from build123d import *

# Parameters (mm, degrees)
SKETCH_1_R          = 1.3
SKETCH_1_W          = 7.4992
SKETCH_1_H          = 3.0001
SKETCH_1_W_2        = 4.9995
EXTRUDE_1_DEPTH     = 3
SKETCH_2_R          = 1.6
CUT_EXTRUDE_1_DEPTH = 57.708942736


with BuildPart() as part:
    # 草图1 → 凸台-拉伸1 (new body)
    with BuildSketch(Plane(origin=(0, 0, 0), x_dir=(-1, 0, 0), z_dir=(0, 0, -1))):
        with BuildLine():
            Line((-30.618171933, 0), (49.343510787, 0))
            ThreePointArc((49.343510787, 0), (55.343510787, 6), (49.343510787, 12))
            Line((49.343510787, 12), (-30.618171933, 12))
            ThreePointArc((-30.618171933, 12), (-36.618171933, 6), (-30.618171933, 0))
        make_face()
        with Locations(Location((49.343510787, 6, 0), (0, 0, 180))):
            Circle(SKETCH_1_R, mode=Mode.SUBTRACT)
        with Locations(Location((1.379286828, 6.00015, 0), (0, 0, 180))):
            Circle(SKETCH_1_R, mode=Mode.SUBTRACT)
        with Locations(Location((-30.611606698, 6.0001, 0), (0, 0, 180))):
            Circle(SKETCH_1_R, mode=Mode.SUBTRACT)
        with Locations((35.628693302, 5.99945)):
            Rectangle(SKETCH_1_W, SKETCH_1_H, mode=Mode.SUBTRACT)
        with Locations((-18.121556698, 5.99945)):
            Rectangle(SKETCH_1_W_2, SKETCH_1_H, mode=Mode.SUBTRACT)
    extrude(amount=-EXTRUDE_1_DEPTH)

    # 草图2 → 切除-拉伸1 (cut, through all)
    with BuildSketch(Plane.XY.offset(3)):
        with Locations((-49.343510787, 6)):
            Circle(SKETCH_2_R)
        with Locations((-1.379286828, 6.00015)):
            Circle(SKETCH_2_R)
    extrude(amount=-CUT_EXTRUDE_1_DEPTH, mode=Mode.SUBTRACT)


solid = part.part
Read the model definition and answer for the solid it produces. Units are mm, in the model's axes. A direction names the side the tool comes from. Coordinates: 2 decimals unless noted, no trailing zeros. Loops run counter-clockwise (first coordinate to the right, second up) from the corner with the lowest first, then second, coordinate; pieces in that order, holes last. Notation, with made-up numbers: (24.5, 7) -> (36.5, 7) arc R16 ccw to (36.5, 19) -> close; hole circle Ø10 at (52.5, 15.25). An arc over 180 degrees is marked (long way). Answer in a Markdown table with one row per item.
Item 1: For a pull along Y with two mould halves and no side action, classify faces 3 (the flat face through (20.621, 6, 1)), 4 (the cylindrical face through (36.617, 6.132, 1.479)), 5 (the flat face through (-10, 12, 1)) as released by +Y, released by -Y, zero draft, split by the parting line, or undercut.
Returned:
| item | result |
|---|---|
| face 3 | undercut |
| face 4 | split by the parting line |
| face 5 | released by +Y |
Item 2: A cutting plane is placed at B-B on z = 0.75. Determine the outline of the cut face in (x, y).
Returned:
| item | result |
|---|---|
| outline | (-49.34, 0) -> (30.62, 0) arc R6 ccw to (30.62, 12) -> (-49.34, 12) arc R6 ccw to start; hole circle Ø3.2 at (-49.34, 6); hole (-39.38, 4.5) -> (-31.88, 4.5) -> (-31.88, 7.5) -> (-39.38, 7.5) -> close; hole circle Ø3.2 at (-1.38, 6); hole (15.62, 4.5) -> (20.62, 4.5) -> (20.62, 7.5) -> (15.62, 7.5) -> close; hole circle Ø2.6 at (30.61, 6) |
Item 3: Straight lines are drawn through the part: line 1 along X through (y, z) = (5.75, 0.95); line 2 along X through (y, z) = (5, 0.2); line 3 along Y through (x, z) = (-37.5, 1.8). For each, find the intervals that lie inside material, in ascending order. Write a range as [from, to].
Returned:
| item | result |
|---|---|
| line 1 | x = [-55.34, -50.92], [-47.76, -39.38], [-31.88, -2.96], [0.2, 15.62], [20.62, 29.34], [31.89, 36.61] |
| line 2 | x = [-55.26, -50.59], [-48.09, -39.38], [-31.88, -2.63], [-0.13, 15.62], [20.62, 29.78], [31.44, 36.53] |
| line 3 | y = [0, 4.5], [7.5, 12] |
Item 4: This flat-tipped pin is pushed along its axis until it touches: P1, Ø1.5, axis at y = 5.5, z = 1.5, coming from the -X side. Where does it stop, or does it pass through?
Returned:
| item | result |
|---|---|
| P1 | stops at x = -55.34 |
Item 5: For faces 1 (the cylindrical face through (-55.342, 5.868, 1.479)), 2 (the flat face through (-36, 7.5, 1)), determine the directions among +Z, -Z, +X, -X, +Y, -Y from which every point of the face is accessible in a straight line to the end or side of a thin tool.
Returned:
| item | result |
|---|---|
| face 1 | +Z, -Z, -X |
| face 2 | +Z, -Z |
Item 6: A cutting plane is placed at A-A on x = -37. Determine the outline of the cut face in (y, z).
Returned:
| item | result |
|---|---|
| outline | (0, 0) -> (4.5, 0) -> (4.5, 3) -> (0, 3) -> close; (7.5, 0) -> (12, 0) -> (12, 3) -> (7.5, 3) -> close |
Item 7: A cutting plane is placed at C-C on y = 1. Determine the outline of the cut face in (x, z), plus the area to 3 significant figures.
Returned:
| item | result |
|---|---|
| outline | (-52.66, 0) -> (33.93, 0) -> (33.93, 3) -> (-52.66, 3) -> close |
| area | 260 mm^2 |
